```python
from build123d import *

# Parameters (mm, degrees)
BOSS_EXTRUDE2_DEPTH             = 30
CUT_EXTRUDE1_DEPTH              = 55.53264752
CUT_EXTRUDE1_DEPTH_BACK         = 55.53264752
SKETCH3_W                       = 22
SKETCH3_H                       = 30.310889132
BOSS_EXTRUDE3_REACH             = 56.533
SKETCH4_W                       = 4
SKETCH4_H                       = 4
BOSS_EXTRUDE3_DIRECTION_2_REACH = 56.533


with BuildPart() as part:
    # Sketch2 → Boss-Extrude2 (new body)
    with BuildSketch(Plane(origin=(0, 0, 0), x_dir=(0, 0, -1), z_dir=(1, 0, 0))):
        Polygon((-2.5, 0), (2.5, 0), (24.618802154, 38.310889132), (20, 38.310889132), (0.190598923, 4), (-0.190598923, 4), (-20, 38.310889132), (-24.618802154, 38.310889132), align=None)
    extrude(amount=BOSS_EXTRUDE2_DEPTH)

    # Sketch3 → Cut-Extrude1 (cut, two sides: drawn at the far end of the back side and taken through both)
    with BuildSketch(Plane.XY.offset(-CUT_EXTRUDE1_DEPTH_BACK)):
        with Locations((15, 19.155444566)):
            Rectangle(SKETCH3_W, SKETCH3_H)
    extrude(amount=CUT_EXTRUDE1_DEPTH + CUT_EXTRUDE1_DEPTH_BACK, mode=Mode.SUBTRACT)

    # Boss-Extrude3: up to this plane
    boss_extrude3_end = Plane(origin=(30, 4, 0.190598923), z_dir=(0, -0.49999999999999795, 0.8660254037844398))
    # Sketch4 → Boss-Extrude3 (add, up to the surface)
    with BuildSketch(Plane.XY, mode=Mode.PRIVATE) as boss_extrude3_sk1:
        with Locations((2, 36.310889132)):
            Rectangle(SKETCH4_W, SKETCH4_H)
    boss_extrude3_tool1 = split(extrude(boss_extrude3_sk1.sketch, amount=BOSS_EXTRUDE3_REACH, mode=Mode.PRIVATE), bisect_by=boss_extrude3_end, keep=Keep.BOTH, mode=Mode.PRIVATE)
    add(boss_extrude3_tool1.solids().sort_by_distance((2, 36.310889, 0))[0])
    # Sketch4 → Boss-Extrude3 (add, up to the surface)
    with BuildSketch(Plane.XY, mode=Mode.PRIVATE) as boss_extrude3_sk2:
        with Locations((28, 36.310889132)):
            Rectangle(SKETCH4_W, SKETCH4_H)
    boss_extrude3_tool2 = split(extrude(boss_extrude3_sk2.sketch, amount=BOSS_EXTRUDE3_REACH, mode=Mode.PRIVATE), bisect_by=boss_extrude3_end, keep=Keep.BOTH, mode=Mode.PRIVATE)
    add(boss_extrude3_tool2.solids().sort_by_distance((28, 36.310889, 0))[0])

    # Boss-Extrude3 direction 2: up to this plane
    boss_extrude3_direction_2_end = Plane(origin=(30, 38.310889132, -20), z_dir=(0, -0.49999999999999756, -0.8660254037844402))
    # Sketch4 → Boss-Extrude3 direction 2 (add, up to the surface)
    with BuildSketch(Plane.XY, mode=Mode.PRIVATE) as boss_extrude3_direction_2_sk1:
        with Locations((2, 36.310889132)):
            Rectangle(SKETCH4_W, SKETCH4_H)
    boss_extrude3_direction_2_tool1 = split(extrude(boss_extrude3_direction_2_sk1.sketch, amount=-BOSS_EXTRUDE3_DIRECTION_2_REACH, mode=Mode.PRIVATE), bisect_by=boss_extrude3_direction_2_end, keep=Keep.BOTH, mode=Mode.PRIVATE)
    add(boss_extrude3_direction_2_tool1.solids().sort_by_distance((2, 36.310889, 0))[0])
    # Sketch4 → Boss-Extrude3 direction 2 (add, up to the surface)
    with BuildSketch(Plane.XY, mode=Mode.PRIVATE) as boss_extrude3_direction_2_sk2:
        with Locations((28, 36.310889132)):
            Rectangle(SKETCH4_W, SKETCH4_H)
    boss_extrude3_direction_2_tool2 = split(extrude(boss_extrude3_direction_2_sk2.sketch, amount=-BOSS_EXTRUDE3_DIRECTION_2_REACH, mode=Mode.PRIVATE), bisect_by=boss_extrude3_direction_2_end, keep=Keep.BOTH, mode=Mode.PRIVATE)
    add(boss_extrude3_direction_2_tool2.solids().sort_by_distance((28, 36.310889, 0))[0])


solid = part.part
```
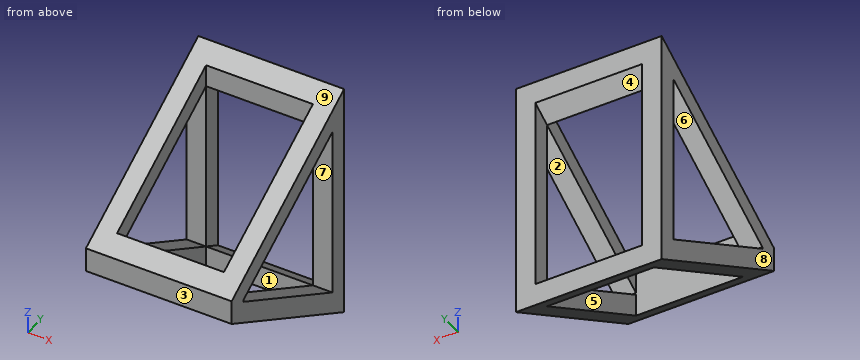
Part model, mm, in its own coordinate system. Face numbers are marked on the shaded views. A direction names the side the tool comes from. Give positions to 0.01 mm unless a question says otherwise; leave off trailing zeros. Order: outer loops, then holes, each group sorted by start corner. A loop starts at its lowest first (then second) coordinate and runs counter-clockwise, first axis right, second up. Notation, with made-up numbers: M -4,-34 L 35,-34 A8 ccw 35,-30 Z; hole C -34.5,37 d4. An arc over 180 degrees is marked long. Use a Markdown table: item, result. Add a question column.
(1) Saw through at B-B, the plane x = 2.25. Give the cut face in (y, z).
(2) Saw through at A-A, the plane x = 10. Give the cut face in (y, z).
(3) 3-axis set-ups, long thin cutter, end or side, ignore diameter. For the marked faces 1, 2, 3, 4 and 5: which of +Z, -Z, +X, -X, +Y, -Y reach the whole face in a straight line?
(4) Saw through at C-C, the plane z = -10.5. Give the cut face in (x, y), and give its area (3 significant figures).
(5) Saw through at D-D, the plane y = 25. Give the cut face in (x, z), and give its area (3 significant figures).
(6) Probe line 1 along X through (y, z) = (35, 12); line 2 along Y through (x, z) = (22.25, -22); line 3 along Y through (x, z) = (14.75, 1). List the from-to ranges inside material, lowest first. Write a range as [from, to].
(7) Drop flat-ended pins along their axis: P1, Ø3.5, axis at x = 12, z = 21, coming from the -Y side; P2, Ø5, axis at x = 21, z = -5.5, coming from the +Y side. Give the stop position or say it passes through.
(8) Mould opens along Z. For the marked faces 6, 7, 8 and 9 say: +Z half, -Z half, draft (parallel to the pull), parting line (faces both ways), or undercut.
Answer key:
| question | item | result |
|---|---|---|
| 1 | outline | M 0,-2.5 L 38.31,-24.62 L 38.31,24.62 L 0,2.5 Z; hole M 4,-0.19 L 34.31,-17.69 L 34.31,17.69 L 4,0.19 Z |
| 2 | outline | M 0,-2.5 L 4,-4.81 L 4,4.81 L 0,2.5 Z; M 34.31,-22.31 L 38.31,-24.62 L 38.31,-20 L 34.31,-17.69 Z; M 34.31,17.69 L 38.31,20 L 38.31,24.62 L 34.31,22.31 Z |
| 3 | face 1 | +Z, -Z, -Y |
| 3 | face 2 | +X, -X |
| 3 | face 3 | +Z, -Z, +X, -X, -Y |
| 3 | face 4 | +Y |
| 3 | face 5 | +Z, -Z |
| 4 | outline | M 0,13.86 L 4,13.86 L 4,21.86 L 0,21.86 Z; M 0,34.31 L 4,34.31 L 4,38.31 L 0,38.31 Z; M 26,13.86 L 30,13.86 L 30,21.86 L 26,21.86 Z; M 26,34.31 L 30,34.31 L 30,38.31 L 26,38.31 Z |
| 4 | area | 96.0 mm^2 |
| 5 | outline | M 0,-16.93 L 4,-16.93 L 4,-12.31 L 0,-12.31 Z; M 0,12.31 L 4,12.31 L 4,16.93 L 0,16.93 Z; M 26,-16.93 L 30,-16.93 L 30,-12.31 L 26,-12.31 Z; M 26,12.31 L 30,12.31 L 30,16.93 L 26,16.93 Z |
| 5 | area | 73.9 mm^2 |
| 6 | line 1 | [0, 4], [26, 30] |
| 6 | line 2 | [34.31, 38.31] |
| 6 | line 3 | [0, 4] |
| 7 | P1 | y = 34.31 |
| 7 | P2 | y = 4 |
| 8 | face 6 | undercut |
| 8 | face 7 | undercut |
| 8 | face 8 | draft |
| 8 | face 9 | +Z half |
